Here's how the part is built. I have some questions about the finished solid (model axes, mm). Round coordinates to 2 decimals unless told otherwise and drop trailing zeros. Order: outer loops, then holes, each group sorted by start corner. A loop starts at its lowest first (then second) coordinate and runs counter-clockwise, first axis right, second up. Notation, with made-up numbers: (54, -35.5) - (106, -35.5) arc R16 ccw to (106, -8.5) - close; hole circle Ø10 at (45, -13.75). An arc over 180 degrees is marked (long way). Answer as a JSON object with one key per item and string values.
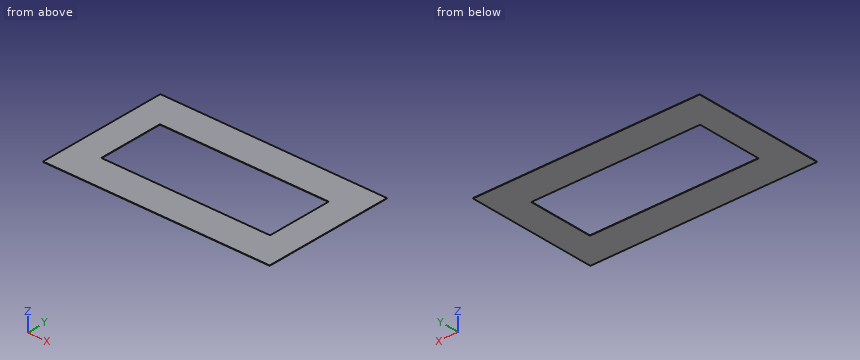
Autodesk Inventor part; units mm, degrees
ref_plane "YZ Plane" through (0, 0, 0) normal (1, 0, 0) x (0, 1, 0)
ref_plane "XZ Plane" through (0, 0, 0) normal (0, 1, 0) x (-1, 0, 0)
ref_plane "XY Plane" through (0, 0, 0) normal (0, 0, 1) x (1, 0, 0)
sketch "Sketch1" plane through (0, 0, 0) normal (0, 0, 1) x (1, 0, 0)
  line L0 (-920.75, -533.4) -> (920.75, -533.4)
  line L1 (920.75, -533.4) -> (920.75, 533.4)
  line L2 (920.75, 533.4) -> (-920.75, 533.4)
  line L3 (-920.75, 533.4) -> (-920.75, -533.4)
  line L4 (-920.75, -533.4) -> (920.75, 533.4) construction
  line L5 (920.75, -533.4) -> (-920.75, 533.4) construction
  point P0 (0, 0)
  dimension "d0" = 1841.5
  dimension "d1" = 1066.8
extrude "Extrusion1" add sketch "Sketch1" against normal blind 3.175
sketch "Sketch2" plane through (0, 0, 0) normal (0, 0, 1) x (1, 0, 0)
  line L0 (-920.75, -533.4) -> (920.75, -533.4)
  line L1 (920.75, -533.4) -> (920.75, 533.4)
  line L2 (920.75, 533.4) -> (-920.75, 533.4)
  line L3 (-920.75, 533.4) -> (-920.75, -533.4)
  line L4 (-685.8, -266.7) -> (685.8, -266.7)
  line L5 (685.8, -266.7) -> (685.8, 266.7)
  line L6 (685.8, 266.7) -> (-685.8, 266.7)
  line L7 (-685.8, 266.7) -> (-685.8, -266.7)
  point P0 (0, 0)
  dimension "d4" = 234.95
  dimension "d5" = 266.7
  dimension "d6" = 234.95
  dimension "d7" = 266.7
extrude "Extrusion2" cut sketch "Sketch2" against normal through all contours L7 L6 L5 L4
properties part number "GE-13011B" material "Polyethylene, High Density"
1. For P1, Ø10, axis at x = -672, y = 282.5, coming from the +Z side, with a flat end and sliding along its axis, tell me the tip position at first contact or that it passes through.
Responses:
{"P1": "z = 0"}
2. Imagine slicing it at B-B (z = -2). List the corners of the cut face in (x, y) for me.
Responses:
{"outline": "(-920.75, -533.4) - (920.75, -533.4) - (920.75, 533.4) - (-920.75, 533.4) - close; hole (-685.8, -266.7) - (685.8, -266.7) - (685.8, 266.7) - (-685.8, 266.7) - close"}
3. Imagine slicing it at A-A (y = -97). List the corners of the cut face in (x, z) for me (3 decimals).
Responses:
{"outline": "(-920.75, -3.175) - (-685.8, -3.175) - (-685.8, 0) - (-920.75, 0) - close; (685.8, -3.175) - (920.75, -3.175) - (920.75, 0) - (685.8, 0) - close"}
4. If I drill on L1, parallel to X at y = -235, z = -2.8; L2, parallel to Y at x = 141, z = -1.3, over which ranges is the centre line in solid material (lowest first)? Write a range as [from, to].
Responses:
{"L1": "[-920.75, -685.8], [685.8, 920.75]", "L2": "[-533.4, -266.7], [266.7, 533.4]"}
5. Imagine slicing it at C-C (x = -81). List the corners of the cut face in (y, z) for me (3 decimals), plus the area to 3 significant figures.
Responses:
{"outline": "(-533.4, -3.175) - (-266.7, -3.175) - (-266.7, 0) - (-533.4, 0) - close; (266.7, -3.175) - (533.4, -3.175) - (533.4, 0) - (266.7, 0) - close", "area": "1,690 mm2"}
